```python
from build123d import *

# Parameters (mm, degrees)
SKETCH2_R           = 2.6
RESISTOR_BODY_DEPTH = 16.2
LEAD1_PROFILE_R     = 0.4
SKETCH6_R           = 0.4
LEAD2_DEPTH         = 5


with BuildPart() as part:
    # Sketch2 → Resistor Body (new body)
    with BuildSketch(Plane.XY):
        Circle(SKETCH2_R)
    extrude(amount=RESISTOR_BODY_DEPTH)

    # Lead1: sweep along a path in Lead1 Path
    with BuildLine(Plane(origin=(0, 0, 0), x_dir=(1, 0, 0), z_dir=(0, 1, 0))) as lead1_path:
        Line((0, -16.2), (0, -18.2))
        ThreePointArc((0, -18.2), (0.585786438, -19.614213562), (2, -20.2))
        Line((2, -20.2), (3, -20.2))
        ThreePointArc((3, -20.2), (4.414213562, -19.614213562), (5, -18.2))
        Line((5, -18.2), (5, 5))
    # Lead1 Profile → Lead1 (sweep)
    with BuildSketch(Plane(origin=(0, 0, 16.2), x_dir=(-1, 0, 0), z_dir=(0, 0, 1))):
        Circle(LEAD1_PROFILE_R)
    sweep(path=lead1_path.line)

    # Sketch6 → Lead2 (add)
    with BuildSketch(Plane(origin=(0, 0, 0), x_dir=(1, 0, 0), z_dir=(0, 0, -1))):
        Circle(SKETCH6_R)
    extrude(amount=LEAD2_DEPTH)


solid = part.part
```
Part model, mm, in its own coordinate system. Round coordinates to 2 decimals unless told otherwise and drop trailing zeros. Loops run counter-clockwise (first coordinate to the right, second up) from the corner with the lowest first, then second, coordinate; pieces in that order, holes last. Notation, with made-up numbers: (47.5, -1) -> (58.5, -1) arc R35 cw to (58.5, 34) -> close; hole circle Ø8 at (14.5, 38). An arc over 180 degrees is marked (long way). Use one line per item in the form item = value. Start each with the question number.
Item 1: Band-saw the part on B-B (y = 0). List the corners of the cut face in (x, z).
Item 2: Drop flat-ended pins along their axis: pin 1 Ø1.5 at (y, z) = (1.5, 3) entering from -X; pin 2 Ø2 at (x, y) = (2, 0.5) entering from -Z. Give the stop position or say it passes through.
Item 3: Band-saw the part on D-D (y = -1.3). List the corners of the cut face in (x, z).
Item 4: Band-saw the part on C-C (x = -1). List the corners of the cut face in (y, z).
Item 5: Drill centre lines: line 1 along Z through (x, y) = (-0.25, 2.2); line 2 along Y through (x, z) = (-2, 15.5); line 3 along X through (y, z) = (-1.9, 5.5). Where is each one in solid material? Low to high.
Item 6: Band-saw the part on A-A (z = 1.5). List the corners of the cut face in (x, y), plus the area to 3 significant figures.
Data:
q1.outline = (-2.6, 0) -> (-0.4, 0) -> (-0.4, -5) -> (0.4, -5) -> (0.4, 0) -> (2.6, 0) -> (2.6, 16.2) -> (0.4, 16.2) -> (0.4, 18.2) arc R1.6 cw to (2, 19.8) -> (3, 19.8) arc R1.6 cw to (4.6, 18.2) -> (4.6, -5) -> (5.4, -5) -> (5.4, 18.2) arc R2.4 ccw to (3, 20.6) -> (2, 20.6) arc R2.4 ccw to (-0.4, 18.2) -> (-0.4, 16.2) -> (-2.6, 16.2) -> close
q2.pin_1 = -2.49
q2.pin_2 = 0
q3.outline = (-2.25, 0) -> (2.25, 0) -> (2.25, 16.2) -> (-2.25, 16.2) -> close
q4.outline = (-2.4, 0) -> (2.4, 0) -> (2.4, 16.2) -> (-2.4, 16.2) -> close
q5.line_1 = 0 to 16.2
q5.line_2 = -1.66 to 1.66
q5.line_3 = -1.77 to 1.77
q6.outline = circle Ø5.2 at (0, 0); circle Ø0.8 at (5, 0)
q6.area = 21.7 mm^2
